from build123d import *

# Parameters (mm, degrees)
SKETCH2_W           = 13
SKETCH2_H           = 23
SKETCH2_R           = 2.2
BOSS_EXTRUDE1_DEPTH = 10
SKETCH5_W           = 5
SKETCH5_H           = 23
BOSS_EXTRUDE2_DEPTH = 2.5
SKETCH6_W           = 5
SKETCH6_H           = 23
BOSS_EXTRUDE3_DEPTH = 7.5
CUT_EXTRUDE2_DEPTH  = 153.496625691
SKETCH8_W           = 13
SKETCH8_H           = 23
SKETCH8_R           = 2.2
BOSS_EXTRUDE4_DEPTH = 5


with BuildPart() as part:
    # Sketch2 → Boss-Extrude1 (new body)
    with BuildSketch(Plane.XY):
        with Locations((-27, -139.600035894)):
            Rectangle(SKETCH2_W, SKETCH2_H)
        with Locations((-27, -144.300035894)):
            Circle(SKETCH2_R, mode=Mode.SUBTRACT)
        with Locations((-27, -134.300035894)):
            Circle(SKETCH2_R, mode=Mode.SUBTRACT)
    extrude(amount=BOSS_EXTRUDE1_DEPTH)

    # Sketch5 → Boss-Extrude2 (add)
    with BuildSketch(Plane(origin=(0, 0, 0), x_dir=(-1, 0, 0), z_dir=(0, 0, -1))):
        with Locations((18, -139.600035894)):
            Rectangle(SKETCH5_W, SKETCH5_H)
        with Locations((36, -139.600035894)):
            Rectangle(SKETCH5_W, SKETCH5_H)
    extrude(amount=-BOSS_EXTRUDE2_DEPTH)

    # Sketch6 → Boss-Extrude3 (add)
    with BuildSketch(Plane(origin=(0, 0, 0), x_dir=(-1, 0, 0), z_dir=(0, 0, -1))):
        with Locations((18, -139.600035894)):
            Rectangle(SKETCH6_W, SKETCH6_H)
        with Locations((36, -139.600035894)):
            Rectangle(SKETCH6_W, SKETCH6_H)
    extrude(amount=BOSS_EXTRUDE3_DEPTH)

    # Sketch7 → Cut-Extrude2 (cut, through all)
    with BuildSketch(Plane(origin=(-20.5, 0, 0), x_dir=(0, 0, -1), z_dir=(1, 0, 0))):
        with BuildLine():
            ThreePointArc((-6.25, -137.400035894), (-8.45, -139.600035894), (-6.25, -141.800035894))
            Line((-6.25, -141.800035894), (-6.25, -137.400035894))
        make_face()
        with BuildLine():
            Line((-6.25, -137.400035894), (-6.25, -141.800035894))
            ThreePointArc((-6.25, -141.800035894), (-4.694365081, -141.155670812), (-4.05, -139.600035894))
            ThreePointArc((-4.05, -139.600035894), (-4.694365081, -138.044400975), (-6.25, -137.400035894))
        make_face()
    extrude(amount=-CUT_EXTRUDE2_DEPTH, mode=Mode.SUBTRACT)

    # Sketch8 → Boss-Extrude4 (add)
    with BuildSketch(Plane.XY.offset(10)):
        with Locations((-27, -139.600035894)):
            Rectangle(SKETCH8_W, SKETCH8_H)
        with Locations((-27, -134.300035894)):
            Circle(SKETCH8_R, mode=Mode.SUBTRACT)
        with Locations((-27, -144.300035894)):
            Circle(SKETCH8_R, mode=Mode.SUBTRACT)
    extrude(amount=BOSS_EXTRUDE4_DEPTH)


solid = part.part
The model under review builds one solid part; all positions refer to its coordinate system, in mm. A direction names the side the tool comes from. Round coordinates to 2 decimals unless told otherwise and drop trailing zeros. Order: outer loops, then holes, each group sorted by start corner. A loop starts at its lowest first (then second) coordinate and runs counter-clockwise, first axis right, second up. Notation, with made-up numbers: (-30, 27.5) -> (-6, 27.5) arc R16 cw to (-6, 36.5) -> close; hole circle Ø7 at (12, -29). An arc over 180 degrees is marked (long way). Write item = value, one per line. Start each with the question number.
Item 1: Clearance check with flat-ended pins moving along their axes: pin 1 Ø5.5 at (x, y) = (-36.5, -134.5) entering from +Z; pin 2 Ø10 at (y, z) = (-136.5, 8.5) entering from +X; pin 3 Ø7 at (x, y) = (-27, -144.3) entering from -Z. State where each tip first meets the part, or that it passes through.
Item 2: Consider section D-D on x = -30.75. Write out the cut boundary in (y, z).
Item 3: Consider section A-A on x = -27. Write out the cut boundary in (y, z).
Item 4: For line 1 along Y through (x, z) = (-27, 9); line 2 along X through (y, z) = (-144.5, -3.5); line 3 along Y through (x, z) = (-27, 6.5), list the stretches that pass through material, from the lowest coordinate up.
Item 5: Mouldability with a two-part tool opening along X and no side actions: class faces 1 (the face through (-38.5, -140, -3)), 2 (the face through (-20.5, -140, -4)), 3 (the face through (-18, -139, -7.5)) as released by +X, released by -X, zero draft, split by the parting line, or undercut.
Item 6: Consider section C-C on y = -133.25. Write out the cut boundary in (x, z), plus the area to 3 significant figures.
Item 7: For faces 4 (the face through (-20.5, -140, 9)), 5 (the face through (-33.5, -140, 9)), 6 (the face through (-33.5, -140, -4)), list the 3-axis set-ups (+Z, -Z, +X, -X, +Y, -Y) from which the entire face can be reached by the end or side of a thin tool; tool diameter is ignored.
Item 8: Consider section B-B on z = 5. Write out the cut boundary in (x, y), plus the area to 3 significant figures.
Conclusion:
q1.pin_1 = 2.5
q1.pin_2 = -20.5
q1.pin_3 = 0
q2.outline = (-151.1, 0) -> (-128.1, 0) -> (-128.1, 15) -> (-151.1, 15) -> close; hole circle Ø4.4 at (-139.6, 6.25)
q3.outline = (-151.1, 0) -> (-146.5, 0) -> (-146.5, 15) -> (-151.1, 15) -> close; (-142.1, 0) -> (-136.5, 0) -> (-136.5, 15) -> (-142.1, 15) -> close; (-132.1, 0) -> (-128.1, 0) -> (-128.1, 15) -> (-132.1, 15) -> close; hole circle Ø4.4 at (-139.6, 6.25)
q4.line_1 = -151.1 to -146.5, -142.1 to -136.5, -132.1 to -128.1
q4.line_2 = -38.5 to -33.5, -20.5 to -15.5
q4.line_3 = -151.1 to -146.5, -142.1 to -141.79, -137.41 to -136.5, -132.1 to -128.1
q5.face_1 = released by -X
q5.face_2 = undercut
q5.face_3 = zero draft
q6.outline = (-38.5, -7.5) -> (-33.5, -7.5) -> (-33.5, 0) -> (-28.93, 0) -> (-28.93, 15) -> (-33.5, 15) -> (-33.5, 2.5) -> (-38.5, 2.5) -> close; (-25.07, 0) -> (-20.5, 0) -> (-20.5, -7.5) -> (-15.5, -7.5) -> (-15.5, 2.5) -> (-20.5, 2.5) -> (-20.5, 15) -> (-25.07, 15) -> close
q6.area = 237 mm2
q7.face_4 = +Z, +X, +Y, -Y
q7.face_5 = +Z, -X, +Y, -Y
q7.face_6 = -Z, +Y, -Y
q8.outline = (-33.5, -151.1) -> (-20.5, -151.1) -> (-20.5, -141.41) -> (-33.5, -141.41) -> close; (-33.5, -137.79) -> (-20.5, -137.79) -> (-20.5, -128.1) -> (-33.5, -128.1) -> close; hole circle Ø4.4 at (-27, -144.3); hole circle Ø4.4 at (-27, -134.3)
q8.area = 222 mm2
